```python
from build123d import *

# Parameters (mm, degrees)
SKETCH1_W           = 292.1
SKETCH1_H           = 438.15
SKETCH1_R           = 7
SKETCH1_R_2         = 14.2875
BOSS_EXTRUDE1_DEPTH = 4.7625
SKETCH2_R           = 14.2875
CUT_EXTRUDE3_DEPTH  = 10.668


with BuildPart() as part:
    # Sketch1 → Boss-Extrude1 (new body)
    with BuildSketch(Plane.XY):
        with Locations((146.05, -219.075)):
            Rectangle(SKETCH1_W, SKETCH1_H)
        with Locations(Location((101.925695163, -306.813385495, 0), (0, 0, 180))):
            Circle(SKETCH1_R, mode=Mode.SUBTRACT)
        with Locations(Location((64.374426387, -313.256382727, 0), (0, 0, 180))):
            Circle(SKETCH1_R, mode=Mode.SUBTRACT)
        with Locations(Location((66.914426387, -356.944382727, 0), (0, 0, 180))):
            Circle(SKETCH1_R_2, mode=Mode.SUBTRACT)
        with Locations(Location((117.714426387, -363.294382727, 0), (0, 0, 180))):
            Circle(SKETCH1_R_2, mode=Mode.SUBTRACT)
        with Locations(Location((168.514426387, -369.644382727, 0), (0, 0, 180))):
            Circle(SKETCH1_R_2, mode=Mode.SUBTRACT)
        with Locations(Location((219.314426387, -375.994382727, 0), (0, 0, 180))):
            Circle(SKETCH1_R_2, mode=Mode.SUBTRACT)
        with Locations(Location((270.114426387, -382.344382727, 0), (0, 0, 180))):
            Circle(SKETCH1_R_2, mode=Mode.SUBTRACT)
    extrude(amount=BOSS_EXTRUDE1_DEPTH)

    # Sketch2 → Cut-Extrude3 (cut)
    with BuildSketch(Plane.XY.offset(4.7625)):
        with Locations((270.114426387, -191.844382727)):
            Circle(SKETCH2_R)
    extrude(amount=-CUT_EXTRUDE3_DEPTH, mode=Mode.SUBTRACT)


solid = part.part
```
Verification items for the finished model (mm, model axes). Round coordinates to 2 decimals unless told otherwise and drop trailing zeros. Loops run counter-clockwise (first coordinate to the right, second up) from the corner with the lowest first, then second, coordinate; pieces in that order, holes last. Notation, with made-up numbers: (-5.75, 9) -> (2.25, 9) arc R17 cw to (2.25, 35) -> close; hole circle Ø7 at (-13, 32.25). An arc over 180 degrees is marked (long way). Answer as a JSON object with one key per item and string values.
Q1. Section check B-B (z = 2.2). State how many separate pieces and enclosed holes the cut face has, then the cut area to 3 significant figures.
Data:
{"separate pieces": "1", "enclosed holes": "8", "area": "124,000 mm2"}
Q2. Go/stop test with a flat-tipped pin: P1, Ø23, axis at x = 270.11, y = -382.34, coming from the +Z side. Record where the tip stops, or that it passes through.
Data:
{"P1": "passes through"}
Q3. Scan lines: line 1 (Y direction, x = 273, z = 1.5); line 2 (Y direction, x = 76.5, z = 0.2); line 3 (X direction, y = -191.5, z = 2.45). Record each from-to range of solid material in increasing order. Write a range as from..to.
Data:
{"line 1": "y = -438.15..-396.34, -368.35..-205.84, -177.85..0", "line 2": "y = -438.15..-367.54, -346.35..0", "line 3": "x = 0..255.83, 284.4..292.1"}
Q4. Section check C-C (x = 262). Record the boundary of the cut face in (y, z).
Data:
{"outline": "(-438.15, 0) -> (-394.1, 0) -> (-394.1, 4.76) -> (-438.15, 4.76) -> close; (-370.58, 0) -> (-203.6, 0) -> (-203.6, 4.76) -> (-370.58, 4.76) -> close; (-180.08, 0) -> (0, 0) -> (0, 4.76) -> (-180.08, 4.76) -> close"}
Q5. Section check D-D (x = 222). Record the boundary of the cut face in (y, z), then the cut area to 3 significant figures.
Data:
{"outline": "(-438.15, 0) -> (-390.03, 0) -> (-390.03, 4.76) -> (-438.15, 4.76) -> close; (-361.96, 0) -> (0, 0) -> (0, 4.76) -> (-361.96, 4.76) -> close", "area": "1,950 mm2"}
Q6. Section check A-A (x = 119). Record the boundary of the cut face in (y, z), then the cut area to 3 significant figures.
Data:
{"outline": "(-438.15, 0) -> (-377.52, 0) -> (-377.52, 4.76) -> (-438.15, 4.76) -> close; (-349.06, 0) -> (0, 0) -> (0, 4.76) -> (-349.06, 4.76) -> close", "area": "1,950 mm2"}
Q7. Draft check along X on faces 1 (the cylindrical face through (103.44, -299.98, 2.35)), 2 (the cylindrical face through (65.286, -320.197, 2.348)), 3 (the flat face through (144, -216, 0)). Enter one of: pulls with the +X half, pulls with the -X half, needs draft (parallel to the pull), parting line crosses it, or undercut.
Data:
{"face 1": "undercut", "face 2": "undercut", "face 3": "needs draft"}
